For this review, use the dimensioned drawing (mm, ordinates from the lowest corner) and the shaded views. Coordinates: 2 decimals unless noted, no trailing zeros. Write each loop counter-clockwise with the first axis right and the second up, starting at its lowest first coordinate (ties: lowest second). Pieces come first, ordered by that corner, then holes. Notation, with made-up numbers: (81.25, -37) -> (120.25, -37) arc R27 ccw to (120.25, -20) -> close; hole circle Ø8 at (4.25, 46). An arc over 180 degrees is marked (long way). Put each result on its own line as item: value. Start each with the question number.
Item 1: Consider section B-B on y = 4. Give the boundary of the cut face in (x, z).
Item 2: Consider section C-C on z = 0.8. Give the boundary of the cut face in (x, y).
Item 3: To check wall thickness, follow L1, parallel to Y at x = 22, z = 0.45; L2, parallel to Y at x = 14, z = 0.65; L3, parallel to X at y = 5.75, z = 0.75. State the ranges of each line that lie inside material, in increasing order.
Item 4: Consider section A-A on x = 14. Give the boundary of the cut face in (y, z).
Item 5: Consider section D-D on x = 32. Give the boundary of the cut face in (y, z).
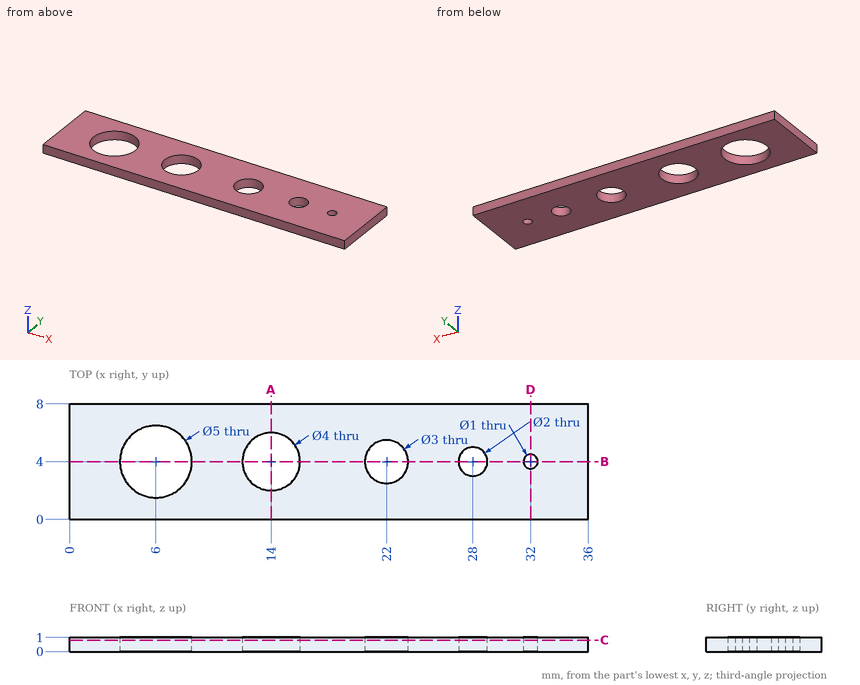
Return value:
1. outline: (0, 0) -> (3.5, 0) -> (3.5, 1) -> (0, 1) -> close; (8.5, 0) -> (12, 0) -> (12, 1) -> (8.5, 1) -> close; (16, 0) -> (20.5, 0) -> (20.5, 1) -> (16, 1) -> close; (23.5, 0) -> (27, 0) -> (27, 1) -> (23.5, 1) -> close; (29, 0) -> (31.5, 0) -> (31.5, 1) -> (29, 1) -> close; (32.5, 0) -> (36, 0) -> (36, 1) -> (32.5, 1) -> close
2. outline: (0, 0) -> (36, 0) -> (36, 8) -> (0, 8) -> close; hole circle Ø5 at (6, 4); hole circle Ø4 at (14, 4); hole circle Ø3 at (22, 4); hole circle Ø2 at (28, 4); hole circle Ø1 at (32, 4)
3. L1: 0 to 2.5, 5.5 to 8
3. L2: 0 to 2, 6 to 8
3. L3: 0 to 4.21, 7.79 to 13.03, 14.97 to 36
4. outline: (0, 0) -> (2, 0) -> (2, 1) -> (0, 1) -> close; (6, 0) -> (8, 0) -> (8, 1) -> (6, 1) -> close
5. outline: (0, 0) -> (3.5, 0) -> (3.5, 1) -> (0, 1) -> close; (4.5, 0) -> (8, 0) -> (8, 1) -> (4.5, 1) -> close
